The listing builds one solid part. Answer for the finished solid, in the listing's coordinates (mm). A direction names the side the tool comes from. Coordinates: 2 decimals unless noted, no trailing zeros. Order: outer loops, then holes, each group sorted by start corner. A loop starts at its lowest first (then second) coordinate and runs counter-clockwise, first axis right, second up. Notation, with made-up numbers: (-4, 82) - (46, 82) arc R16 ccw to (46, 87) - close; hole circle Ø6 at (77, 22). An arc over 180 degrees is marked (long way). Use a Markdown table: item, result. Add a question column.
Item 1: Flat-ended cylindrical pins translate along their axes: P1, Ø3, axis at y = -6, z = -118, coming from the -X side; P2, Ø1.5, axis at x = -144, y = -3.5, coming from the -Z side; P3, Ø2, axis at y = -4.5, z = -57, coming from the -X side. Find the tip coordinate at first contact, or state that the pin passes through.
Item 2: The part is cut by section C-C, the plane y = -8. State how many separate pieces and enclosed holes the cut face has, then the cut area to 3 significant figures.
Item 3: For faces 1 (the flat face through (25, -5, -65)), 2 (the cylindrical face through (-7, -5, 7)), 3 (the flat face through (-97, -5, -33.5)), determine the directions among +Z, -Z, +X, -X, +Y, -Y from which every point of the face is accessible in a straight line to the end or side of a thin tool.
Item 4: The part is cut by section A-A, the plane x = 0. Give the vertices of the cut face in (y, z).
Item 5: The part is cut by section B-B, the plane z = -113. Give the vertices of the cut face in (x, y), then the cut area to 3 significant figures.
Item 6: The part is cut by section D-D, the plane x = -92.5. Give the vertices of the cut face in (y, z), then the cut area to 3 significant figures.
Item 7: The mould has two halves that part along X. Classify faces 4 (the cylindrical face through (-23.574, -4.93, -142.8)), 5 (the cylindrical face through (7, -5, 7)), 6 (the flat face through (-46, -10, -28)): released by +X, released by -X, zero draft, split by the parting line, or undercut.
Item 8: Find the intervals of material crossed by line 1 along Z through (x, y) = (-145, -5.5); line 2 along X through (y, z) = (-7.5, -135.5); line 3 along Z through (x, y) = (-15, -7.5), in increasing order.
from build123d import *

# Parameters (mm, degrees)
F0_R     = 2
F1_DEPTH = 10


with BuildPart() as f1:
    # F0 (on Front) → F1 (new body)
    with BuildSketch(Plane.XZ):
        with BuildLine():
            ThreePointArc((-141, -30), (-139.974874, -32.474874), (-137.5, -33.5))
            Line((-137.5, -33.5), (-55, -33.5))
            ThreePointArc((-55, -33.5), (-33.786797, -42.286797), (-25, -63.5))
            Line((-25, -63.5), (-25, -139.304042))
            ThreePointArc((-25, -139.304042), (-23.535534, -142.839575), (-20, -144.304042))
            Line((-20, -144.304042), (20, -144.304042))
            ThreePointArc((20, -144.304042), (23.535534, -142.839575), (25, -139.304042))
            Line((25, -139.304042), (25, 10.695958))
            ThreePointArc((25, 10.695958), (23.535534, 14.231492), (20, 15.695958))
            Line((20, 15.695958), (10.995904, 15.695958))
            ThreePointArc((10.995904, 15.695958), (8.52103, 14.670832), (7.495904, 12.195958))
            Line((7.495904, 12.195958), (7.495904, 9.943808))
            ThreePointArc((7.495904, 9.943808), (7.153343, 7.442143), (5.999985, 5.195938))
            Line((5.999985, 5.195938), (5.999985, 3.709538))
            ThreePointArc((5.999985, 3.709538), (5.614844, 1.580886), (4.499852, -0.272836))
            Line((4.499852, -0.272836), (4.499852, -2.267552))
            ThreePointArc((4.499852, -2.267552), (-0.005832, -6.804038), (-4.499742, -2.255887))
            Line((-4.499742, -2.255887), (-4.499742, -0.272961))
            ThreePointArc((-4.499742, -0.272961), (-5.616003, 1.583966), (-5.999966, 3.716286))
            Line((-5.999966, 3.716286), (-5.999966, 5.195912))
            ThreePointArc((-5.999966, 5.195912), (-7.177791, 7.521258), (-7.488602, 10.109288))
            Line((-7.488602, 10.109288), (-7.441414, 12.113578))
            ThreePointArc((-7.441414, 12.113578), (-8.436614, 14.641533), (-10.940444, 15.695958))
            Line((-10.940444, 15.695958), (-150, 15.695958))
            ThreePointArc((-150, 15.695958), (-153.535534, 14.231492), (-155, 10.695958))
            Line((-155, 10.695958), (-155, -30))
            ThreePointArc((-155, -30), (-153.974874, -32.474874), (-151.5, -33.5))
            ThreePointArc((-151.5, -33.5), (-149.025126, -32.474874), (-148, -30))
            Line((-148, -30), (-148, -28.5))
            ThreePointArc((-148, -28.5), (-147.414214, -27.085787), (-146, -26.5))
            Line((-146, -26.5), (-143, -26.5))
            ThreePointArc((-143, -26.5), (-141.585786, -27.085787), (-141, -28.5))
            Line((-141, -28.5), (-141, -30))
        make_face()
        with Locations((-15, -134.304042)):
            Circle(F0_R, mode=Mode.SUBTRACT)
        with Locations((0, -134.304042)):
            Circle(F0_R, mode=Mode.SUBTRACT)
        with Locations((15, -134.304042)):
            Circle(F0_R, mode=Mode.SUBTRACT)
        with Locations((-145, -9.304042)):
            Circle(F0_R, mode=Mode.SUBTRACT)
        with Locations((-145, 5.695958)):
            Circle(F0_R, mode=Mode.SUBTRACT)
    extrude(amount=F1_DEPTH)


solid = f1.part
Solution:
| question | item | result |
|---|---|---|
| 1 | P1 | stops at x = -25 |
| 1 | P2 | stops at z = -26.5 |
| 1 | P3 | stops at x = -25.95 |
| 2 | separate pieces | 1 |
| 2 | enclosed holes | 5 |
| 2 | area | 14,200 mm2 |
| 3 | face 1 | +Z, -Z, +X, +Y, -Y |
| 3 | face 2 | +Y, -Y |
| 3 | face 3 | -Z, -X, +Y, -Y |
| 4 | outline | (-10, -144.3) - (0, -144.3) - (0, -136.3) - (-10, -136.3) - close; (-10, -132.3) - (0, -132.3) - (0, -6.8) - (-10, -6.8) - close |
| 5 | outline | (-25, -10) - (25, -10) - (25, 0) - (-25, 0) - close |
| 5 | area | 500 mm2 |
| 6 | outline | (-10, -33.5) - (0, -33.5) - (0, 15.7) - (-10, 15.7) - close |
| 6 | area | 492 mm2 |
| 7 | face 4 | released by -X |
| 7 | face 5 | undercut |
| 7 | face 6 | zero draft |
| 8 | line 1 | z = -26.5 to -11.3, -7.3 to 3.7, 7.7 to 15.7 |
| 8 | line 2 | x = -25 to -16.6, -13.4 to -1.6, 1.6 to 13.4, 16.6 to 25 |
| 8 | line 3 | z = -144.3 to -136.3, -132.3 to 15.7 |
